The model under review builds one solid part; all positions refer to its coordinate system, in mm. A direction names the side the tool comes from. Coordinates: 2 decimals unless noted, no trailing zeros. Loops run counter-clockwise (first coordinate to the right, second up) from the corner with the lowest first, then second, coordinate; pieces in that order, holes last. Notation, with made-up numbers: (80.25, 34.5) - (84.25, 34.5) arc R29 ccw to (84.25, 64.5) - close; hole circle Ø2 at (69, -35). An arc over 180 degrees is marked (long way). Answer in a Markdown table with one row per item. Add a question column.
(1) For P1, Ø2, axis at x = 0.5, y = -2, coming from the -Z side; P2, Ø2.5, axis at x = 0, y = 0, coming from the -Z side, all flat-tipped, find the tip position at first contact; note any pin that passes through.
(2) Mouldability with a two-part tool opening along X and no side actions: class faces 3 (the flat face through (3, 0, 3)), 4 (the cylindrical face through (0, -1, 3)), 5 (the flat face through (1.5, 0, 1)), 6 (the flat face through (0, 3, 3)) as +X half, -X half, draft (parallel to the pull), parting line (faces both ways), or undercut.
(3) For line 1 along Y through (x, z) = (0, 2.5); line 2 along X through (y, z) = (-0.3, 1.45); line 3 along Y through (x, z) = (-0.35, 2.05), list the stretches that pass through material, from the lowest coordinate up.
(4) We need section A-A on x = 0. Write out the cut boundary in (y, z), plus the area to 3 significant figures.
(5) We need section D-D on y = -1.15. Write out the cut boundary in (x, z), plus the area to 3 significant figures.
(6) We need section C-C on z = 4.65. Write out the cut boundary in (x, y), plus the area to 3 significant figures.
(7) Machinability: for faces 1 (the flat face through (0, 1.5, 1)), 2 (the flat face through (-1, 1, 5.328)), which of the approach directions +Z, -Z, +X, -X, +Y, -Y give a long, thin tool a straight path to every point of the face, cutting with its end or side? Answer none if there is none.
from build123d import *

# Parameters (mm, degrees)
F0_W     = 6
F0_H     = 6
F0_W_2   = 3
F0_H_2   = 3
F0_R     = 1
F2_DEPTH = 5.328427
F3_DEPTH = 1.5
F4_R     = 1


with BuildPart() as f2:
    # F0 (on Top) → F2 (new body, through all)
    with BuildSketch(Plane.XY):
        Rectangle(F0_W, F0_H)
        Rectangle(F0_W_2, F0_H_2, mode=Mode.SUBTRACT)
        Rectangle(F0_W_2, F0_H_2)
        Circle(F0_R, mode=Mode.SUBTRACT)
    extrude(amount=F2_DEPTH)

    # F0 (on Top) → F3 (cut)
    with BuildSketch(Plane.XY):
        Rectangle(F0_W_2, F0_H_2)
        Circle(F0_R, mode=Mode.SUBTRACT)
    extrude(amount=F3_DEPTH, mode=Mode.SUBTRACT)

    # F4
    f4_edges = [f2.edges().sort_by_distance(p)[0] for p in [
        (-3, -3, 2.664214),
        (3, -3, 2.664214),
        (3, 3, 2.664214),
        (-3, 3, 2.664214),
    ]]
    fillet(f4_edges, radius=F4_R)


solid = f2.part
Outcome:
| question | item | result |
|---|---|---|
| 1 | P1 | z = 0 |
| 1 | P2 | z = 1.5 |
| 2 | face 3 | +X half |
| 2 | face 4 | undercut |
| 2 | face 5 | undercut |
| 2 | face 6 | draft |
| 3 | line 1 | -3 to -1, 1 to 3 |
| 3 | line 2 | -3 to -1.5, 1.5 to 3 |
| 3 | line 3 | -3 to -0.94, 0.94 to 3 |
| 4 | outline | (-3, 0) - (-1.5, 0) - (-1.5, 1.5) - (-1, 1.5) - (-1, 5.33) - (-3, 5.33) - close; (1, 1.5) - (1.5, 1.5) - (1.5, 0) - (3, 0) - (3, 5.33) - (1, 5.33) - close |
| 4 | area | 19.8 mm² |
| 5 | outline | (-3, 0) - (-1.5, 0) - (-1.5, 1.5) - (1.5, 1.5) - (1.5, 0) - (3, 0) - (3, 5.33) - (-3, 5.33) - close |
| 5 | area | 27.5 mm² |
| 6 | outline | (-3, -2) arc R1 ccw to (-2, -3) - (2, -3) arc R1 ccw to (3, -2) - (3, 2) arc R1 ccw to (2, 3) - (-2, 3) arc R1 ccw to (-3, 2) - close; hole circle Ø2 at (0, 0) |
| 6 | area | 32.0 mm² |
| 7 | face 1 | -Z |
| 7 | face 2 | +Z, +X, -X, +Y, -Y |
